from build123d import *

# Parameters (mm, degrees)
SKETCH1_R           = 18.85
SKETCH1_R_2         = 10
SKETCH1_R_3         = 4
BOSS_EXTRUDE1_DEPTH = 11
SKETCH1_3_R         = 20.05
SKETCH1_3_R_2       = 18.85
BOSS_EXTRUDE2_DEPTH = 1.5
BOSS_EXTRUDE3_START = 11
SKETCH1_4_R         = 20.05
SKETCH1_4_R_2       = 18.85
SKETCH1_4_R_3       = 10
SKETCH1_4_R_4       = 4
BOSS_EXTRUDE3_DEPTH = 1.5
SKETCH1_5_R         = 10
SKETCH1_5_R_2       = 4
BOSS_EXTRUDE4_DEPTH = 18


with BuildPart() as part:
    # Sketch1 → Boss-Extrude1 (new body)
    with BuildSketch(Plane.XY):
        Circle(SKETCH1_R)
        Circle(SKETCH1_R_2, mode=Mode.SUBTRACT)
        Circle(SKETCH1_R_2)
        Circle(SKETCH1_R_3, mode=Mode.SUBTRACT)
    extrude(amount=BOSS_EXTRUDE1_DEPTH)

    # Sketch1_3 → Boss-Extrude2 (add)
    with BuildSketch(Plane.XY):
        Circle(SKETCH1_3_R)
        Circle(SKETCH1_3_R_2, mode=Mode.SUBTRACT)
    extrude(amount=BOSS_EXTRUDE2_DEPTH)

    # Sketch1_4 → Boss-Extrude3 (add)
    with BuildSketch(Plane.XY.offset(BOSS_EXTRUDE3_START)):
        Circle(SKETCH1_4_R)
        Circle(SKETCH1_4_R_2, mode=Mode.SUBTRACT)
        Circle(SKETCH1_4_R_3)
        Circle(SKETCH1_4_R_4, mode=Mode.SUBTRACT)
    extrude(amount=-BOSS_EXTRUDE3_DEPTH)

    # Sketch1_5 → Boss-Extrude4 (add)
    with BuildSketch(Plane.XY):
        Circle(SKETCH1_5_R)
        Circle(SKETCH1_5_R_2, mode=Mode.SUBTRACT)
    extrude(amount=BOSS_EXTRUDE4_DEPTH)


solid = part.part
Could you check a few things on this model? Use its own coordinates, in mm. A direction names the side the tool comes from. Coordinates: 2 decimals unless noted, no trailing zeros. Order: outer loops, then holes, each group sorted by start corner. A loop starts at its lowest first (then second) coordinate and runs counter-clockwise, first axis right, second up. Notation, with made-up numbers: (24.5, 75) -> (46.5, 75) arc R27 ccw to (46.5, 108) -> close; hole circle Ø9 at (8.5, -38.5). An arc over 180 degrees is marked (long way). One line per item, written item: value. Start each with the question number.
1) Imagine slicing it at A-A on x = 0. List the corners of the cut face in (y, z) for me, plus the area to 3 significant figures.
2) Imagine slicing it at D-D on x = 12.5. List the corners of the cut face in (y, z) for me.
3) Imagine slicing it at C-C on z = 2.5. List the corners of the cut face in (x, y) for me, plus the area to 3 significant figures.
4) If I drill on L1, parallel to Y at x = 0, z = 11.25; L2, parallel to Y at x = 0, z = 6.25; L3, parallel to Z at x = -14, y = 6, over which ranges is the centre line in solid material (lowest first)? Write a range as [from, to].
5) Which directions (+Z, -Z, +X, -X, +Y, -Y) give clear straight access to the entire face, cutting with the end or side of a thin tool? Please do faces 4 (the flat face through (-0.1, -4.3, 18)), 5 (the flat face through (-9, 5, 11)), 6 (the cylindrical face through (-4.1, -18.4, 5.4)).
6) We'd pull the mould along Y, two halves only. Please class faces 1 (the cylindrical face through (-0.867, -3.905, 8.874)), 2 (the cylindrical face through (-15.91, -12.2, 0.74)), 3 (the flat face through (15, -12, 9.5)): +Y half, -Y half, draft (parallel to the pull), parting line (faces both ways), or undercut.
7) I'm going to push flat-ended pins straight in: pin 1 (5 mm diameter, centred on x = -3, z = 4.5, fed in from +Y); pin 2 (1 mm diameter, centred on y = -8, z = 14, fed in from -X); pin 3 (6 mm diameter, centred on x = 4.5, y = -11.5, fed in from +Z); pin 4 (2 mm diameter, centred on x = -16, z = 3.5, fed in from +Y). Where does each tip first touch, or does it pass through?
Answer list:
1. outline: (-20.05, 0) -> (-4, 0) -> (-4, 18) -> (-10, 18) -> (-10, 11) -> (-20.05, 11) -> (-20.05, 9.5) -> (-18.85, 9.5) -> (-18.85, 1.5) -> (-20.05, 1.5) -> close; (4, 0) -> (20.05, 0) -> (20.05, 1.5) -> (18.85, 1.5) -> (18.85, 9.5) -> (20.05, 9.5) -> (20.05, 11) -> (10, 11) -> (10, 18) -> (4, 18) -> close
1. area: 418 mm2
2. outline: (-15.68, 0) -> (15.68, 0) -> (15.68, 1.5) -> (14.11, 1.5) -> (14.11, 9.5) -> (15.68, 9.5) -> (15.68, 11) -> (-15.68, 11) -> (-15.68, 9.5) -> (-14.11, 9.5) -> (-14.11, 1.5) -> (-15.68, 1.5) -> close
3. outline: circle Ø37.7 at (0, 0); hole circle Ø8 at (0, 0)
3. area: 1,070 mm2
4. L1: y = [-10, -4], [4, 10]
4. L2: y = [-18.85, -4], [4, 18.85]
4. L3: z = [0, 11]
5. face 4: +Z, +X, -X, +Y, -Y
5. face 5: +Z
5. face 6: none
6. face 1: undercut
6. face 2: parting line
6. face 3: draft
7. pin 1: stops at y = 18.84
7. pin 2: stops at x = -6.61
7. pin 3: stops at z = 18
7. pin 4: stops at y = 11.42
